from build123d import *

# Parameters (mm, degrees)
CROQUIS1_R              = 6.35
SALIENTE_EXTRUIR1_DEPTH = 12.7
REDONDEO2_R             = 2
CROQUIS2_R              = 1.27
CORTAR_EXTRUIR1_DEPTH   = 12.7
CROQUIS4_R              = 3.175
SALIENTE_EXTRUIR2_DEPTH = 12.7
CROQUIS3_R              = 1.5875
CORTAR_EXTRUIR2_DEPTH   = 27.881433379
CROQUIS5_W              = 1.5875
CROQUIS5_H              = 31.254771719
CORTAR_EXTRUIR3_DEPTH   = 12.7


with BuildPart() as part:
    # Croquis1 → Saliente-Extruir1 (new body)
    with BuildSketch(Plane.XY):
        Circle(CROQUIS1_R)
    extrude(amount=SALIENTE_EXTRUIR1_DEPTH)

    # Redondeo2
    redondeo2_edges = [part.edges().sort_by_distance(p)[0] for p in [
        (-6.35, 0, 0),
    ]]
    fillet(redondeo2_edges, radius=REDONDEO2_R)

    # Croquis2 → Cortar-Extruir1 (cut)
    with BuildSketch(Plane.XY.offset(12.7)):
        with Locations((-6.35, 0)):
            Circle(CROQUIS2_R)
        with Locations((-5.499261314, 3.175)):
            Circle(CROQUIS2_R)
        with Locations((-3.175, 5.499261314)):
            Circle(CROQUIS2_R)
        with Locations((0, 6.35)):
            Circle(CROQUIS2_R)
        with Locations((3.175, 5.499261314)):
            Circle(CROQUIS2_R)
        with Locations((5.499261314, 3.175)):
            Circle(CROQUIS2_R)
        with Locations((6.35, 0)):
            Circle(CROQUIS2_R)
        with Locations((5.499261314, -3.175)):
            Circle(CROQUIS2_R)
        with Locations((3.175, -5.499261314)):
            Circle(CROQUIS2_R)
        with Locations((0, -6.35)):
            Circle(CROQUIS2_R)
        with Locations((-3.175, -5.499261314)):
            Circle(CROQUIS2_R)
        with Locations((-5.499261314, -3.175)):
            Circle(CROQUIS2_R)
    extrude(amount=-CORTAR_EXTRUIR1_DEPTH, mode=Mode.SUBTRACT)

    # Croquis4 → Saliente-Extruir2 (add)
    with BuildSketch(Plane.XY.offset(12.7)):
        Circle(CROQUIS4_R)
    extrude(amount=SALIENTE_EXTRUIR2_DEPTH)

    # Croquis3 → Cortar-Extruir2 (cut, through all)
    with BuildSketch(Plane(origin=(0, 0, 0), x_dir=(-1, 0, 0), z_dir=(0, 0, -1))):
        Circle(CROQUIS3_R)
    extrude(amount=-CORTAR_EXTRUIR2_DEPTH, mode=Mode.SUBTRACT)

    # Croquis5 → Cortar-Extruir3 (cut)
    with BuildSketch(Plane(origin=(0, 0, 0), x_dir=(1, 0, 0), z_dir=(0, 1, 0))):
        with Locations((0, -15.62738586)):
            Rectangle(CROQUIS5_W, CROQUIS5_H)
    extrude(amount=CORTAR_EXTRUIR3_DEPTH, mode=Mode.SUBTRACT)


solid = part.part
Model file for the job. Use its own axes, mm. A direction names the side the tool comes from. Round coordinates to 2 decimals unless told otherwise and drop trailing zeros. Write each question's results on one line, items separated by ' | '. Start each with the question number.
(1) Drop flat-ended pins along their axis: pin 1 (5 mm diameter, centred on x = 2, z = 20.5, fed in from -Y) (3 decimals); pin 2 (5 mm diameter, centred on x = 0.5, z = 22, fed in from +Y); pin 3 (1 mm diameter, centred on x = -3.5, z = 9, fed in from -Y); pin 4 (4 mm diameter, centred on x = 0, y = 0, fed in from -Z). Give the stop position or say it passes through.
(2) Probe probe 1 along X at (y, z) = (3.5, 11); probe 2 along X at (y, z) = (1, 12.75); probe 3 along Y at (x, z) = (-5.5, 4.75) (3 decimals). List the from-to ranges inside material, lowest first. Write a range as from..to.
(3) Two-plate mould, pull along X, no slides. Class faces 1 (the face through (0, -2, 0)), 2 (the face through (0.794, 3, 10)), 3 (the face through (-0.128, -3.172, 18.961)): pulls with the +X half, pulls with the -X half, needs draft (parallel to the pull), parting line crosses it, or undercut.
(4) Which spindle directions (+Z, -Z, +X, -X, +Y, -Y) get a long thin tool onto all of the face, cutting with end or side? Do faces 4 (the face through (-0.794, 3, 10)), 5 (the face through (-3, 3, 12.7)), 6 (the face through (0.058, -1.586, 12.522)). Say none if no direction does.
Established:
1) pin 1: stops at y = -3.175 | pin 2: stops at y = 3.07 | pin 3: stops at y = -4.53 | pin 4: stops at z = 0
2) probe 1: x = -4.27..-0.79, 0.79..4.27 | probe 2: x = -3.01..-1.23, 1.23..3.01 | probe 3: y = -1.905..-0.944, 0.944..1.905
3) face 1: needs draft | face 2: undercut | face 3: parting line crosses it
4) face 4: +Z, -Z, +Y | face 5: +Z | face 6: +Z, -Z
